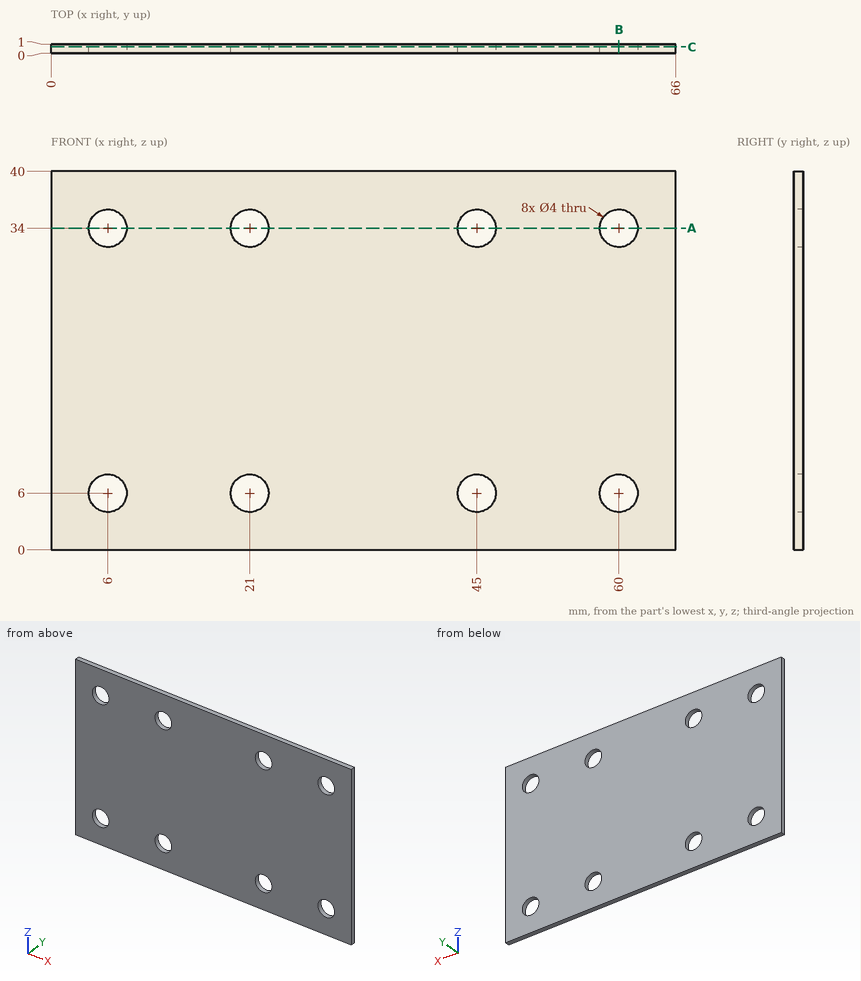
Geometry: see drawing. Coordinates: mm, zero at the bounding-box minimum. Coordinates: 2 decimals unless noted, no trailing zeros. Loops run counter-clockwise (first coordinate to the right, second up) from the corner with the lowest first, then second, coordinate; pieces in that order, holes last. Notation, with made-up numbers: (-37.5, 65.5) - (-8.5, 65.5) arc R13 ccw to (-8.5, 76.5) - close; hole circle Ø3 at (32, 45). An arc over 180 degrees is marked (long way). Put each result on its own line as item: value. Start each with the question number.
Q1. Cut plane B-B, the plane x = 60. Return loops of the section in (y, z), and give its area (3 significant figures).
Q2. Line query: line 1 (Z direction, x = 45, y = 0.35); line 2 (X direction, y = 0.65, z = 35.5); line 3 (Z direction, x = 60.5, y = 0.95). Output: solid intervals per line, ascending.
Q3. Cut plane A-A, the plane z = 34. Return loops of the section in (x, y), and give its area (3 significant figures).
Q4. Pin query (flat end, axial travel): pin 1 Ø8 at (x, z) = (48.5, 35.5) entering from -Y. Return the tip coordinate at first contact, or that it passes through.
Q5. Cut plane C-C, the plane y = 0.7. Give the number of separate pieces and of enclosed holes in the cut face, and give its area (3 significant figures).
Filled sheet:
1. outline: (0, 0) - (1, 0) - (1, 4) - (0, 4) - close; (0, 8) - (1, 8) - (1, 32) - (0, 32) - close; (0, 36) - (1, 36) - (1, 40) - (0, 40) - close
1. area: 32.0 mm²
2. line 1: 0 to 4, 8 to 32, 36 to 40
2. line 2: 0 to 4.68, 7.32 to 19.68, 22.32 to 43.68, 46.32 to 58.68, 61.32 to 66
2. line 3: 0 to 4.06, 7.94 to 32.06, 35.94 to 40
3. outline: (0, 0) - (4, 0) - (4, 1) - (0, 1) - close; (8, 0) - (19, 0) - (19, 1) - (8, 1) - close; (23, 0) - (43, 0) - (43, 1) - (23, 1) - close; (47, 0) - (58, 0) - (58, 1) - (47, 1) - close; (62, 0) - (66, 0) - (66, 1) - (62, 1) - close
3. area: 50.0 mm²
4. pin 1: y = 0
5. separate pieces: 1
5. enclosed holes: 8
5. area: 2,540 mm²
